Geometry check sheet. Reference: the model listing, model coordinates, mm. A direction names the side the tool comes from. Give positions to 0.01 mm unless a question says otherwise; leave off trailing zeros. Write each loop counter-clockwise with the first axis right and the second up, starting at its lowest first coordinate (ties: lowest second). Pieces come first, ordered by that corner, then holes. Notation, with made-up numbers: M 32,-12 L 61,-12 A25 ccw 61,7 Z; hole C -40,17.5 d1. An arc over 180 degrees is marked long. Write each question's results on one line, items separated by ' | '.
Autodesk Inventor part; units mm, degrees
ref_plane "Work Plane1" through (0, -117.4264, 0) normal (0, 0.7071068, -0.7071068) x (1, 0, 0)
ref_plane "YZ Plane" through (0, 0, 0) normal (1, 0, 0) x (0, 1, 0)
ref_plane "XZ Plane" through (0, 0, 0) normal (0, 1, 0) x (-1, 0, 0)
sketch "Sketch1" plane through (0, 0, 0) normal (0, 0, 1) x (1, 0, 0)
  line L0 (130, 75) -> (-130, 75)
  line L1 (-130, 75) -> (-130, -75)
  line L2 (-130, -75) -> (130, -75)
  line L3 (130, -75) -> (130, 75)
  line L4 (130, 75) -> (-130, -75) construction
  line L5 (-130, 75) -> (130, -75) construction
  line L6 (100, 40) -> (-100, 40)
  line L7 (-100, 40) -> (-100, -40)
  line L8 (-100, -40) -> (100, -40)
  line L9 (100, -40) -> (100, 40)
  line L10 (100, 40) -> (-100, -40) construction
  line L11 (-100, 40) -> (100, -40) construction
  point P0 (0, 0)
  point P1 (0, 0)
  point P2 (0, 0)
  point P3 (100, 0)
  point P4 (130, 0)
  dimension "d34" = 200
  dimension "d35" = 80
  dimension "d51" = 30
  dimension "d53" = 30
  dimension "d54" = 35
  dimension "d56" = 150
extrude "Plate1" add sketch "Sketch1" along normal blind 2
sketch "Sketch6" plane through (130, -73.5858, 1.4142) normal (0, -0.7071068, -0.7071068) x (1, 0, 0)
  line L0 (-260, 0) -> (0, 0)
  line L1 (0, 0) -> (0, 60)
  line L2 (0, 60) -> (-260, 60)
  line L3 (-260, 60) -> (-260, 0)
edge flange "Flange2" height 60 angle 45 thickness 2 bend radius 2.75 thickness toward (0, -0.7071068, -0.7071068) relief round relief width 2 relief depth 1 edges at (0, -75, 2) wall of the first edge with corners at (-130, -73.5858, 1.4142) (130, -73.5858, 1.4142) (130, -116.0122, 43.8406) (-130, -116.0122, 43.8406)
bend "Bend2"
corner "Corner2"
sketch "Sketch8" plane through (130, -115.4264, 42.4264) normal (0, -1, 0) x (1, 0, 0)
  line L0 (-260, 0) -> (0, 0)
  line L1 (0, 0) -> (0, 150)
  line L2 (0, 150) -> (-260, 150)
  line L3 (-260, 150) -> (-260, 0)
edge flange "Flange3" height 150 angle 45 thickness 2 bend radius 2.75 thickness toward (0, -1, 0) relief round relief width 2 relief depth 1 edges at (0, -116.0122, 43.8406) wall of the first edge with corners at (-130, -115.4264, 42.4264) (130, -115.4264, 42.4264) (130, -115.4264, 192.4264) (-130, -115.4264, 192.4264)
bend "Bend3"
corner "Corner3"
sketch "Sketch9" plane through (130, -116.0122, 191.0122) normal (0, -0.7071068, 0.7071068) x (1, 0, 0)
  line L0 (-260, 0) -> (0, 0)
  line L1 (0, 0) -> (0, 58.6)
  line L2 (0, 58.6) -> (-260, 58.6)
  line L3 (-260, 58.6) -> (-260, 0)
edge flange "Flange4" height 58.6 angle 45 thickness 2 bend radius 2.75 thickness toward (0, -0.7071068, 0.7071068) relief round relief width 2 relief depth 1 edges at (0, -115.4264, 192.4264) wall of the first edge with corners at (-130, -116.0122, 191.0122) (130, -116.0122, 191.0122) (130, -74.5757, 232.4487) (-130, -74.5757, 232.4487)
bend "Bend4"
corner "Corner4"
sketch "Sketch10" plane through (-130, -117.4264, 44.3939) normal (0, -1, 0) x (1, 0, 0)
  line L0 (260, 146.065) -> (0, 146.065)
  line L1 (0, 0) -> (0, 146.065)
  line L2 (0, 0) -> (260, 0)
  line L3 (260, 146.065) -> (260, 0)
  line L4 (30, 33.0325) -> (230, 33.0325)
  line L5 (230, 33.0325) -> (230, 113.0325)
  line L6 (230, 113.0325) -> (30, 113.0325)
  line L7 (30, 113.0325) -> (30, 33.0325)
  point P0 (130, -44.3939)
  point P1 (30, 73.0325)
  point P2 (0, 73.0325)
  dimension "d77" = 80
  dimension "d78" = 200
  dimension "d79" = 30
extrude "Cut3" cut sketch "Sketch10" against normal blind 2 contours L7 L6 L5 L4
sketch "Sketch11" plane through (0, 0, 0) normal (0, 0, -1) x (-1, 0, 0)
  line L0 (100, -40) -> (-100, -40) construction
  line L1 (-100, -40) -> (-100, 40) construction
  line L2 (-100, 40) -> (100, 40) construction
  line L3 (100, 40) -> (100, -40) construction
  circle A0 centre (0, -53) radius 2.75
  circle A1 centre (0, 53) radius 2.75
  line L4 (-100, 0) -> (100, 0) construction
  point P0 (0, 0)
  dimension "d82" = 106
  dimension "d83" = 5.5
extrude "Cut4" cut sketch "Sketch11" against normal blind 2
pattern_linear "Rectangular Pattern1" count 3 spacing 113 along (1, 0, 0) of "Cut4" first direction both ways yes
ref_plane "Work Plane1" through (0, -117.4264, 0) normal (0, 0.7071068, -0.7071068) x (1, 0, 0)
mirror "Mirror1" about plane through (0, -117.4264, 0) normal (0, 0.7071068, -0.7071068) of "Cut4", "Rectangular Pattern1"
equation "\"d34\" = MAIN_6_central_window_hight"
equation "\"d35\" = MAIN_7_central_window_width"
equation "\"d56\" = Wall_1_width"
equation "\"d77\" = MAIN_7_central_window_width"
equation "\"d78\" = MAIN_6_central_window_hight"
equation "\"d79\" = d53"
equation "\"d80\" = Thickness"
equation "\"d84\" = Thickness"
equation "\"d2\" = Thickness"
equation "\"d36\" = BendReliefWidth"
equation "\"d37\" = BendReliefDepth"
equation "\"d38\" = MinimumRemnant"
equation "\"d39\" = TransitionRadius"
equation "\"d40\" = Wall_2_width"
equation "\"d42\" = BendRadius"
equation "\"d43\" = CornerReliefSize"
equation "\"d44\" = GapSize"
equation "\"d45\" = JacobiRadiusSize"
equation "\"d57\" = BendReliefWidth"
equation "\"d58\" = BendReliefDepth"
equation "\"d59\" = MinimumRemnant"
equation "\"d60\" = TransitionRadius"
equation "\"d61\" = d56"
equation "\"d63\" = BendRadius"
equation "\"d64\" = CornerReliefSize"
equation "\"d65\" = GapSize"
equation "\"d66\" = JacobiRadiusSize"
equation "\"d67\" = BendReliefWidth"
equation "\"d68\" = BendReliefDepth"
equation "\"d69\" = MinimumRemnant"
equation "\"d70\" = TransitionRadius"
equation "\"d71\" = Wall_2_width - 0.7 * Thickness"
equation "\"d73\" = BendRadius"
equation "\"d74\" = CornerReliefSize"
equation "\"d75\" = GapSize"
equation "\"d76\" = JacobiRadiusSize"
equation "\"BendReliefWidth\" = Thickness"
equation "\"BendReliefDepth\" = 0.5 * Thickness"
equation "\"CornerReliefSize\" = 4 * Thickness"
equation "\"MinimumRemnant\" = 2 * Thickness"
equation "\"TransitionRadius\" = BendRadius"
equation "\"JacobiRadiusSize\" = BendRadius"
equation "\"GapSize\" = Thickness"
properties part number "TKS 3554 BOTTOM DS box wall 1" material "Stainless Steel"
Q1. Access from +Z, -Z, +X, -X, +Y, -Y to the whole of each face (thin tool, end or side, straight path). Record for faces 4 (the face through (1.82, -94.52, 22.35)), 5 (the face through (2, -117.426, 167)).
Answer key:
face 4: +X, -X, +Y | face 5: +Z, -Z, +X, -X, -Y
Q2. Section check C-C (y = -15). Enter the section's corners in (x, z).
Answer key:
outline: M -130,0 L -100,0 L -100,2 L -130,2 Z; M 100,0 L 130,0 L 130,2 L 100,2 Z
Q3. Release check for a two-part mould opening along Z. For faces 1 (the face through (-2, -47, 0)), 2 (the face through (1.82, -94.879, 212.146)), 3 (the face through (-2, -47, 2)) record: released by +Z, released by -Z, zero draft, split by the parting line, or undercut.
Answer key:
face 1: released by -Z | face 2: undercut | face 3: released by +Z
Q4. Section check A-A (z = 138). Enter the section's corners in (x, y), then the cut area to 3 significant figures.
Answer key:
outline: M -130,-117.43 L -100,-117.43 L -100,-115.43 L -130,-115.43 Z; M 100,-117.43 L 130,-117.43 L 130,-115.43 L 100,-115.43 Z | area: 120 mm2
Q5. Section check B-B (x = -79). Enter the section's corners in (y, z).
Answer key:
outline: M -117.43,44.39 A4.75 ccw -116.04,41.04 L -76.39,1.39 A4.75 ccw -73.03,0 L -40,0 L -40,2 L -73.03,2 A2.75 cw -74.98,2.81 L -114.62,42.45 A2.75 cw -115.43,44.39 L -115.43,77.43 L -117.43,77.43 Z; M -117.43,157.43 L -115.43,157.43 L -115.43,190.46 A2.75 cw -114.62,192.4 L -74.58,232.45 L -75.99,233.86 L -116.04,193.82 A4.75 ccw -117.43,190.46 Z; M 40,0 L 75,0 L 75,2 L 40,2 Z
Q6. Depth check by flat-ended pin: P1, Ø1.5, axis at x = 103.5, y = 28.5, coming from the +Z side; P2, Ø7, axis at x = 113, y = 53, coming from the -Z side; P3, Ø9, axis at x = 113, z = 170.43, coming from the +Y side; P4, Ø2, axis at x = -92.5, z = 207, coming from the -Y side. Enter the tip coordinate at first touch or a pass-through.
Answer key:
P1: stops at z = 2 | P2: stops at z = 0 | P3: stops at y = -115.43 | P4: stops at y = -103.85
Q7. Material ranges on probe 1 along Z at (x, y) = (0, -116); probe 2 along Z at (x, y) = (113, -116.7); probe 3 along Y at (x, z) = (-64, 161.5), recorded low to high. Write a range as [from, to].
Answer key:
probe 1: z = [41, 61.68], [67.18, 77.43], [157.43, 167.68], [173.18, 193.85] | probe 2: z = [41.87, 61.68], [67.18, 167.68], [173.18, 192.98] | probe 3: y = [-117.43, -115.43]
Q8. Section check D-D (x = 107). Enter the section's corners in (y, z), then the cut area to 3 significant figures.
Answer key:
outline: M -117.43,44.39 A4.75 ccw -116.04,41.04 L -76.39,1.39 A4.75 ccw -73.03,0 L 75,0 L 75,2 L -73.03,2 A2.75 cw -74.98,2.81 L -114.62,42.45 A2.75 cw -115.43,44.39 L -115.43,190.46 A2.75 cw -114.62,192.4 L -74.58,232.45 L -75.99,233.86 L -116.04,193.82 A4.75 ccw -117.43,190.46 Z | area: 831 mm2
